Can you work these out from the model? Positions are in its coordinate system, mm. A direction names the side the tool comes from. Coordinates: 2 decimals unless noted, no trailing zeros. Loops run counter-clockwise (first coordinate to the right, second up) from the corner with the lowest first, then second, coordinate; pieces in that order, holes last. Notation, with made-up numbers: M 28,-4.75 L 39,-4.75 A16 cw 39,9.25 Z; hole C 37.25,84 d11. An arc over 180 degrees is marked long. Answer as a JSON object with one key per item and string values. Group by question number.
Item 1: Suppose I cut it at C-C (x = 19). Write out the boundary of the cut face in (y, z).
Item 2: We'd pull the mould along X, two halves only. Please class faces 3 (the cylindrical face through (11.69, 20.28, 4.97)), 4 (the cylindrical face through (-7.81, 22.33, 1.48)), 5 (the cylindrical face through (19.595, -2.14, 1.479)), 6 (the flat face through (10, 6, 0)): +X half, -X half, draft (parallel to the pull), parting line (faces both ways), or undercut.
Item 3: If I drill on line 1 (Y direction, x = 18.45, z = 1.05); line 2 (Y direction, x = 5.45, z = 2); line 3 (Z direction, x = 2, y = -1), over which ranges is the centre line in solid material (lowest first)?
Item 4: Suppose I cut it at A-A (y = 10.5). Write out the boundary of the cut face in (x, z), then the cut area to 3 significant figures.
Item 5: Suppose I cut it at D-D (y = -2.5). Write out the boundary of the cut face in (x, z).
Item 6: I'm going to push flat-ended pins straight in: pin 1 Ø1.9 at (x, y) = (18.45, 23.5) entering from -Z; pin 2 Ø4 at (y, z) = (7.5, 3.5) entering from -X; pin 3 Ø8 at (x, y) = (17.5, -6) entering from +Z; pin 4 Ø1 at (x, z) = (-1.5, 4) entering from -Y. Where does each tip first touch, or does it pass through?
Item 7: Suppose I cut it at B-B (z = 1). Write out the boundary of the cut face in (x, y).
Item 8: Which directions (+Z, -Z, +X, -X, +Y, -Y) give clear straight access to the entire face, cutting with the end or side of a thin tool? Please do faces 1 (the flat face through (-5, 16, 3)), 2 (the flat face through (10, 6, 7)).
```python
from build123d import *

# Parameters (mm, degrees)
SKETCH_1_R               = 22.5
SKETCH_1_R_2             = 6
SKETCH_1_R_3             = 1.2
EXTRUDE_1_DEPTH          = 3
SKETCH_3_R               = 11.6
SKETCH_3_R_2             = 7.6
EXTRUDE_2_DEPTH          = 4.2
CUT_EXTRUDE_START        = -0.2
SKETCH_4_R               = 11.6
CUT_EXTRUDE_1_DEPTH      = 0.2
SKETCH_5_R               = 7.6
SKETCH_5_R_2             = 6
EXTRUDE_3_DEPTH          = 4
CUT_EXTRUDE_2_DEPTH      = 10
CUT_EXTRUDE_2_DEPTH_BACK = 10


with BuildPart() as part:
    # 草图1 → 凸台-拉伸1 (new body)
    with BuildSketch(Plane.XY):
        with Locations((5.45, 10.5)):
            Circle(SKETCH_1_R)
        with Locations((5.45, 10.5)):
            Circle(SKETCH_1_R_2, mode=Mode.SUBTRACT)
        with Locations((-7.55, -2.5)):
            Circle(SKETCH_1_R_3, mode=Mode.SUBTRACT)
        with Locations((-7.55, 23.5)):
            Circle(SKETCH_1_R_3, mode=Mode.SUBTRACT)
        with Locations((18.45, 23.5)):
            Circle(SKETCH_1_R_3, mode=Mode.SUBTRACT)
        with Locations((18.45, -2.5)):
            Circle(SKETCH_1_R_3, mode=Mode.SUBTRACT)
    extrude(amount=EXTRUDE_1_DEPTH)

    # 草图3 → 凸台-拉伸2 (add)
    with BuildSketch(Plane.XY.offset(3)):
        with Locations((5.45, 10.5)):
            Circle(SKETCH_3_R)
        with Locations((5.45, 10.5)):
            Circle(SKETCH_3_R_2, mode=Mode.SUBTRACT)
    extrude(amount=EXTRUDE_2_DEPTH)

    # 草图4 → 切除-拉伸1 (cut)
    with BuildSketch(Plane.XY.offset(7.2).offset(CUT_EXTRUDE_START)):
        with Locations((5.45, 10.5)):
            Circle(SKETCH_4_R)
    extrude(amount=CUT_EXTRUDE_1_DEPTH, mode=Mode.SUBTRACT)

    # 草图5 → 凸台-拉伸3 (add)
    with BuildSketch(Plane.XY.offset(3)):
        with Locations((5.45, 10.5)):
            Circle(SKETCH_5_R)
        with Locations((5.45, 10.5)):
            Circle(SKETCH_5_R_2, mode=Mode.SUBTRACT)
    extrude(amount=EXTRUDE_3_DEPTH)

    # 草图6 → 切除-拉伸2 (cut, two sides: drawn at the far end of the back side and taken through both)
    with BuildSketch(Plane(origin=(0, 0, 0), x_dir=(1, 0, 0), z_dir=(0, 1, 0)).offset(-CUT_EXTRUDE_2_DEPTH_BACK)):
        with BuildLine():
            ThreePointArc((6.7, -5), (5.556579945, -3.754552002), (4.218174855, -4.787616354))
            Line((4.218174855, -4.787616354), (6.681825145, -5.212383646))
            ThreePointArc((6.681825145, -5.212383646), (6.695447998, -5.106579945), (6.7, -5))
        make_face()
        with BuildLine():
            Line((6.681825145, -5.212383646), (4.218174855, -4.787616354))
            ThreePointArc((4.218174855, -4.787616354), (5.237616354, -6.231825145), (6.681825145, -5.212383646))
        make_face()
    extrude(amount=CUT_EXTRUDE_2_DEPTH + CUT_EXTRUDE_2_DEPTH_BACK, mode=Mode.SUBTRACT)


solid = part.part
```
From the geometry:
{
 "1": {"outline": "M -7.46,0 L -3.57,0 L -3.57,3 L -7.46,3 Z; M -1.43,0 L 22.43,0 L 22.43,3 L -1.43,3 Z; M 24.57,0 L 28.46,0 L 28.46,3 L 24.57,3 Z"},
 "2": {"face 3": "parting line", "face 4": "undercut", "face 5": "undercut", "face 6": "draft"},
 "3": {"line 1": "-7.86 to -3.7, -1.3 to 22.3, 24.7 to 28.86", "line 2": "-12 to 4.5, 16.5 to 33", "line 3": "0 to 3"},
 "4": {"outline": "M -17.05,0 L -0.55,0 L -0.55,7 L -6.15,7 L -6.15,3 L -17.05,3 Z; M 11.45,0 L 27.95,0 L 27.95,3 L 17.05,3 L 17.05,7 L 11.45,7 Z", "area": "144 mm2"},
 "5": {"outline": "M -12.91,0 L -8.75,0 L -8.75,3 L -12.91,3 Z; M -6.35,0 L 17.25,0 L 17.25,3 L -6.35,3 Z; M 19.65,0 L 23.81,0 L 23.81,3 L 19.65,3 Z"},
 "6": {"pin 1": "through", "pin 2": "x = -17.02", "pin 3": "z = 3", "pin 4": "y = 0.86"},
 "7": {"outline": "C 5.45,10.5 d45; hole C -7.55,-2.5 d2.4; hole C -7.55,23.5 d2.4; hole C 5.45,10.5 d12; hole C 18.45,-2.5 d2.4; hole C 18.45,23.5 d2.4"},
 "8": {"face 1": "+Z", "face 2": "+Z, +X, -X, +Y, -Y"}
}
